Read the model definition and answer for the solid it produces. Units are mm, in the model's axes. A direction names the side the tool comes from. Round coordinates to 2 decimals unless told otherwise and drop trailing zeros. Order: outer loops, then holes, each group sorted by start corner. A loop starts at its lowest first (then second) coordinate and runs counter-clockwise, first axis right, second up. Notation, with made-up numbers: (-14, 89.25) -> (27, 89.25) arc R34 ccw to (27, 127.25) -> close; hole circle Ø10 at (13, 34.25). An arc over 180 degrees is marked (long way). One line per item, written item: value. Start each with the question number.
1. Flat-ended cylindrical pins translate along their axes: pin 1 Ø4 at (y, z) = (26, -1) entering from -X; pin 2 Ø12 at (x, z) = (184.5, 12) entering from +Y; pin 3 Ø4 at (x, z) = (38, 32) entering from -Y. Find the tip coordinate at first contact, or state that the pin passes through.
2. The mould has two halves that part along Z. Classify faces 1 (the face through (135.457, -52.886, -6.944)), 2 (the face through (179.7, 20.8, -4.6)), 3 (the face through (267.174, 35, -13)): released by +Z, released by -Z, zero draft, split by the parting line, or undercut.
3. Section A-A (y = 0) is taken. Give the vertices of the cut face in (x, z).
4. For faces 4 (the face through (70.483, -12.999, 41.278)), 5 (the face through (222.95, 15.135, -19.739)), determine the directions among +Z, -Z, +X, -X, +Y, -Y from which every point of the face is accessible in a straight line to the end or side of a thin tool.
5. Section C-C (x = 77.5) is taken. Give the vertices of the cut face in (y, z), then the cut area to 3 significant figures.
6. Consider line 1 (Y direction, x = 92, z = 0); line 2 (Y direction, x = 82, z = 14.5); line 3 (Z direction, x = 97, y = -12). Determine where each line is inside the solid, lowest interval first.
7. Section D-D (x = 240) is taken. Give the vertices of the cut face in (y, z).
from build123d import *


with BuildPart() as part:
    # Sketch1 → Revolve1 (revolve)
    with BuildSketch(Plane.XY, mode=Mode.PRIVATE) as revolve1_sk:
        with BuildLine():
            Line((0, 53.34), (267.174285764, 53.34))
            Line((267.174285764, 53.34), (267.174285764, 36.7237391))
            Line((267.174285764, 36.7237391), (195.627584968, 17.5528584))
            ThreePointArc((195.627584968, 17.5528584), (188.286684173, 17.23234775), (181.498114964, 20.044265185))
            Line((181.498114964, 20.044265185), (152.703069528, 40.206773063))
            ThreePointArc((152.703069528, 40.206773063), (148.071235785, 42.490940687), (142.96691498, 43.2765708))
            Line((142.96691498, 43.2765708), (0, 43.2765708))
            Line((0, 43.2765708), (0, 53.34))
        make_face()
    revolve(revolve1_sk.sketch.rotate(Axis((0, 0, 0), (1, 0, 0)), 90), axis=Axis((0, 0, 0), (1, 0, 0)))


solid = part.part
Answer:
1. pin 1: x = 170.11
1. pin 2: y = 53
1. pin 3: y = -44.1
2. face 1: split by the parting line
2. face 2: undercut
2. face 3: zero draft
3. outline: (0, -53.34) -> (267.17, -53.34) -> (267.17, -36.72) -> (195.63, -17.55) arc R16.97 ccw to (181.5, -20.04) -> (152.7, -40.21) arc R16.97 cw to (142.97, -43.28) -> (0, -43.28) -> close; (0, 43.28) -> (142.97, 43.28) arc R16.97 cw to (152.7, 40.21) -> (181.5, 20.04) arc R16.97 ccw to (195.63, 17.55) -> (267.17, 36.72) -> (267.17, 53.34) -> (0, 53.34) -> close
4. face 4: -X
4. face 5: +X
5. outline: circle Ø106.68 at (0, 0); hole circle Ø86.55 at (0, 0)
5. area: 3,050 mm^2
6. line 1: -53.34 to -43.28, 43.28 to 53.34
6. line 2: -51.33 to -40.78, 40.78 to 51.33
6. line 3: -51.97 to -41.58, 41.58 to 51.97
7. outline: circle Ø106.68 at (0, 0); hole circle Ø58.88 at (0, 0)
